Check sheet for the modelled part. Datum: model origin and axes. Units: mm. Coordinates: 2 decimals unless noted, no trailing zeros. Loops run counter-clockwise (first coordinate to the right, second up) from the corner with the lowest first, then second, coordinate; pieces in that order, holes last.
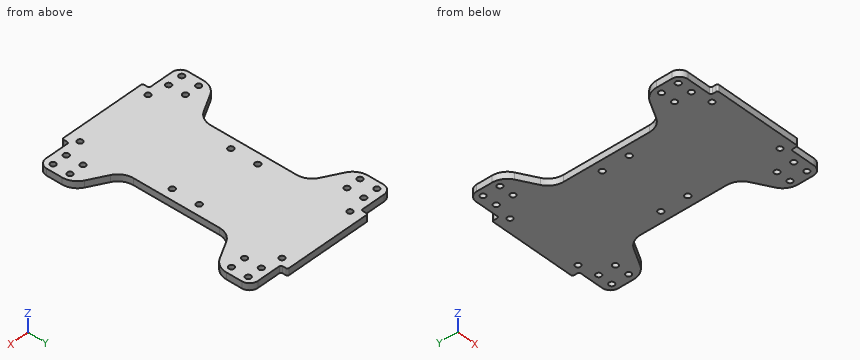
```python
from build123d import *

# Parameters (mm, degrees)
SKETCH1_R           = 1.6
SKETCH1_R_2         = 1.65
BOSS_EXTRUDE1_DEPTH = 4
FILLET2_R           = 10
FILLET3_R           = 5


with BuildPart() as part:
    # Sketch1 → Boss-Extrude1 (new body)
    with BuildSketch(Plane.XY):
        with BuildLine():
            Line((1.40773023, -0.063608297), (20.206941284, -0.063608297))
            ThreePointArc((20.206941284, -0.063608297), (20.914048066, -0.356501516), (21.206941284, -1.063608297))
            Line((21.206941284, -1.063608297), (21.206941284, -3.063608297))
            ThreePointArc((21.206941284, -3.063608297), (21.499834503, -3.770715079), (22.206941284, -4.063608297))
            Line((22.206941284, -4.063608297), (72.208519176, -4.063608297))
            ThreePointArc((72.208519176, -4.063608297), (72.915625957, -3.770715079), (73.208519176, -3.063608297))
            Line((73.208519176, -3.063608297), (73.208519176, -1.063608297))
            ThreePointArc((73.208519176, -1.063608297), (73.501412395, -0.356501516), (74.208519176, -0.063608297))
            Line((74.208519176, -0.063608297), (93.00773023, -0.063608297))
            Line((93.00773023, -0.063608297), (93.00773023, 19.936391703))
            Line((93.00773023, 19.936391703), (72.20773023, 31.430017028))
            Line((72.20773023, 31.430017028), (72.20773023, 94.442766377))
            Line((72.20773023, 94.442766377), (93.00773023, 105.936391703))
            Line((93.00773023, 105.936391703), (93.00773023, 125.936391703))
            Line((93.00773023, 125.936391703), (74.208519176, 125.936391703))
            ThreePointArc((74.208519176, 125.936391703), (73.501412395, 126.229284921), (73.208519176, 126.936391703))
            Line((73.208519176, 126.936391703), (73.208519176, 128.936391703))
            ThreePointArc((73.208519176, 128.936391703), (72.915625957, 129.643498484), (72.208519176, 129.936391703))
            Line((72.208519176, 129.936391703), (22.206941284, 129.936391703))
            ThreePointArc((22.206941284, 129.936391703), (21.499834503, 129.643498484), (21.206941284, 128.936391703))
            Line((21.206941284, 128.936391703), (21.206941284, 126.936391703))
            ThreePointArc((21.206941284, 126.936391703), (20.914048066, 126.229284921), (20.206941284, 125.936391703))
            Line((20.206941284, 125.936391703), (1.40773023, 125.936391703))
            Line((1.40773023, 125.936391703), (1.40773023, 105.936391703))
            Line((1.40773023, 105.936391703), (22.20773023, 94.442766377))
            Line((22.20773023, 94.442766377), (22.20773023, 31.430017028))
            Line((22.20773023, 31.430017028), (1.40773023, 19.936391703))
            Line((1.40773023, 19.936391703), (1.40773023, -0.063608297))
        make_face()
        with Locations((5.55773023, 4.936391703)):
            Circle(SKETCH1_R, mode=Mode.SUBTRACT)
        with Locations((14.05773023, 4.936391703)):
            Circle(SKETCH1_R, mode=Mode.SUBTRACT)
        with Locations((14.05773023, 14.936391703)):
            Circle(SKETCH1_R, mode=Mode.SUBTRACT)
        with Locations((5.55773023, 14.936391703)):
            Circle(SKETCH1_R, mode=Mode.SUBTRACT)
        with Locations((69.208519176, 2.936391703)):
            Circle(SKETCH1_R, mode=Mode.SUBTRACT)
        with Locations((66.20773023, 54.936391703)):
            Circle(SKETCH1_R_2, mode=Mode.SUBTRACT)
        with Locations((88.85773023, 14.936391703)):
            Circle(SKETCH1_R, mode=Mode.SUBTRACT)
        with Locations((80.35773023, 14.936391703)):
            Circle(SKETCH1_R, mode=Mode.SUBTRACT)
        with Locations((80.35773023, 4.936391703)):
            Circle(SKETCH1_R, mode=Mode.SUBTRACT)
        with Locations((88.85773023, 4.936391703)):
            Circle(SKETCH1_R, mode=Mode.SUBTRACT)
        with Locations((28.20773023, 54.936391703)):
            Circle(SKETCH1_R_2, mode=Mode.SUBTRACT)
        with Locations((25.206941284, 2.936391703)):
            Circle(SKETCH1_R, mode=Mode.SUBTRACT)
        with Locations((25.206941284, 122.936391703)):
            Circle(SKETCH1_R, mode=Mode.SUBTRACT)
        with Locations((28.20773023, 70.936391703)):
            Circle(SKETCH1_R_2, mode=Mode.SUBTRACT)
        with Locations((88.85773023, 120.936391703)):
            Circle(SKETCH1_R, mode=Mode.SUBTRACT)
        with Locations((80.35773023, 120.936391703)):
            Circle(SKETCH1_R, mode=Mode.SUBTRACT)
        with Locations((80.35773023, 110.936391703)):
            Circle(SKETCH1_R, mode=Mode.SUBTRACT)
        with Locations((88.85773023, 110.936391703)):
            Circle(SKETCH1_R, mode=Mode.SUBTRACT)
        with Locations((66.20773023, 70.936391703)):
            Circle(SKETCH1_R_2, mode=Mode.SUBTRACT)
        with Locations((69.208519176, 122.936391703)):
            Circle(SKETCH1_R, mode=Mode.SUBTRACT)
        with Locations((5.55773023, 110.936391703)):
            Circle(SKETCH1_R, mode=Mode.SUBTRACT)
        with Locations((14.05773023, 110.936391703)):
            Circle(SKETCH1_R, mode=Mode.SUBTRACT)
        with Locations((14.05773023, 120.936391703)):
            Circle(SKETCH1_R, mode=Mode.SUBTRACT)
        with Locations((5.55773023, 120.936391703)):
            Circle(SKETCH1_R, mode=Mode.SUBTRACT)
    extrude(amount=BOSS_EXTRUDE1_DEPTH)

    # Fillet2
    fillet2_edges = [part.edges().sort_by_distance(p)[0] for p in [
        (1.40773023, 19.936391703, 2),
        (22.20773023, 31.430017028, 2),
        (22.20773023, 94.442766377, 2),
        (1.40773023, 105.936391703, 2),
        (93.00773023, 105.936391703, 2),
        (72.20773023, 94.442766377, 2),
        (72.20773023, 31.430017028, 2),
        (93.00773023, 19.936391703, 2),
    ]]
    fillet(fillet2_edges, radius=FILLET2_R)

    # Fillet3
    fillet3_edges = [part.edges().sort_by_distance(p)[0] for p in [
        (1.40773023, 125.936391703, 2),
        (93.00773023, 125.936391703, 2),
        (93.00773023, -0.063608297, 2),
        (1.40773023, -0.063608297, 2),
    ]]
    fillet(fillet3_edges, radius=FILLET3_R)


solid = part.part
```
1) Section check B-B on z = 3.05. Give the number of separate pieces and of enclosed holes in the cut face, plus the area to 3 significant figures.
Answer sheet:
separate pieces: 1
enclosed holes: 24
area: 8,640 mm2
2) Depth check by flat-ended pin: pin 1 (1 mm diameter, centred on y = -2, z = 2, fed in from -X); pin 2 (5 mm diameter, centred on x = 80.36, y = 14.94, fed in from +Z); pin 3 (1.2 mm diameter, centred on x = 80, z = 3, fed in from +Y). Enter the tip coordinate at first touch or a pass-through.
Answer sheet:
pin 1: stops at x = 21.21
pin 2: stops at z = 4
pin 3: stops at y = 125.94
3) Scan lines: line 1 (X direction, y = 124, z = 2.5); line 2 (X direction, y = 46, z = 0.5); line 3 (Y direction, x = 79.5, z = 2.7). Record each from-to range of solid material in increasing order.
Answer sheet:
line 1: x = 2.46 to 24.01, 26.4 to 68.01, 70.4 to 91.96
line 2: x = 22.21 to 72.21
line 3: y = -0.06 to 3.59, 6.29 to 13.59, 16.29 to 27.4, 98.47 to 109.59, 112.29 to 119.59, 122.29 to 125.94
4) Section check A-A on x = 18.5. Enter the section's corners in (y, z), plus the area to 3 significant figures.
Answer sheet:
outline: (-0.06, 0) - (29.56, 0) - (29.56, 4) - (-0.06, 4) - close; (96.32, 0) - (125.94, 0) - (125.94, 4) - (96.32, 4) - close
area: 237 mm2
